Work out the finished part from the listing and answer in its coordinate system (mm). A direction names the side the tool comes from. Round coordinates to 2 decimals unless told otherwise and drop trailing zeros. Order: outer loops, then holes, each group sorted by start corner. A loop starts at its lowest first (then second) coordinate and runs counter-clockwise, first axis right, second up. Notation, with made-up numbers: (41.5, 30) - (59.5, 30) arc R17 ccw to (59.5, 53) - close; hole circle Ø6 at (-23, 82.25). An arc over 180 degrees is marked (long way). Use one line per item in the form item = value. Start each with the question number.
Q1. The part is cut by section B-B on x = 3.5. Determine the outline of the cut face in (y, z), plus the area to 3 significant figures.
Q2. The part is cut by section D-D on y = 8. Determine the outline of the cut face in (x, z), plus the area to 3 significant figures.
Q3. Given P1, Ø1.3, axis at y = -6.5, z = -16, coming from the -X side; P2, Ø2, axis at x = 13, z = -14.5, coming from the -Y side; P3, Ø2.5, axis at x = 5, y = 6.5, coming from the -Z side, each flat-ended and moving along its own axis, determine where each tip first touches the part or whether it passes through.
Q4. For a pull along X with two mould halves and no side action, classify faces 1 (the flat face through (-1, 1, 18)), 2 (the flat face through (37.42, 3.47, 8.53)), 3 (the cylindrical face through (36.579, 0.76, 14.655)) as +X half, -X half, draft (parallel to the pull), parting line (faces both ways), or undercut.
Q5. The part is cut by section A-A on x = 37.5. Determine the outline of the cut face in (y, z).
Q6. Find the intervals of material crossed by line 1 (X direction, y = 0.85, z = 15.5); line 2 (Z direction, x = -37.5, y = 0.55); line 3 (X direction, y = 4.25, z = 6), in increasing order. Write a range as [from, to].
Q7. Which of the six approach directions +Z, -Z, +X, -X, +Y, -Y give full straight-line access (tool end or side, diameter ignored) to faces 4 (the flat face through (1, 6, -12.3)), 5 (the flat face through (-13, -9, -17.5)), 6 (the flat face through (-35.05, 6, 0)), 7 (the flat face through (0, 6, 12.9))?
Q8. The part is cut by section C-C on z = 2.5. Determine the outline of the cut face in (x, y), plus the area to 3 significant figures.
from build123d import *

# Parameters (mm, degrees)
SCHIZZO1_W                   = 80
SCHIZZO1_H                   = 36
ESTRUSIONE_ESTRUSIONE1_DEPTH = 1.5
SCHIZZO2_R                   = 1.25
TAGLIO_ESTRUSIONE1_DEPTH     = 1.5
ESTRUSIONE_ESTRUSIONE2_DEPTH = 8.6
SCHIZZO3_3_W                 = 71.2
SCHIZZO3_3_H                 = 25.2
ESTRUSIONE_ESTRUSIONE3_DEPTH = 4
SCHIZZO4_W                   = 41
SCHIZZO4_H                   = 2.54
ESTRUSIONE_ESTRUSIONE4_DEPTH = 18


with BuildPart() as part:
    # Schizzo1 → Estrusione-Estrusione1 (new body)
    with BuildSketch(Plane(origin=(0, 0, 0), x_dir=(1, 0, 0), z_dir=(0, 1, 0))):
        Rectangle(SCHIZZO1_W, SCHIZZO1_H)
    extrude(amount=ESTRUSIONE_ESTRUSIONE1_DEPTH)

    # Schizzo2 → Taglio-Estrusione1 (cut)
    with BuildSketch(Plane(origin=(0, 1.5, 0), x_dir=(1, 0, 0), z_dir=(0, 1, 0))):
        with Locations((-37.5, 15.5)):
            Circle(SCHIZZO2_R)
        with Locations((37.5, 15.5)):
            Circle(SCHIZZO2_R)
        with Locations((-37.5, -15.5)):
            Circle(SCHIZZO2_R)
        with Locations((37.5, -15.5)):
            Circle(SCHIZZO2_R)
    extrude(amount=-TAGLIO_ESTRUSIONE1_DEPTH, mode=Mode.SUBTRACT)

    # Schizzo3 → Estrusione-Estrusione2 (add)
    with BuildSketch(Plane(origin=(0, 1.5, 0), x_dir=(1, 0, 0), z_dir=(0, 1, 0))):
        Polygon((36.15, 12.3), (-35.05, 12.3), (-35.05, -12.9), (36.15, -12.9), (36.15, -9.8), (36.15, -0.3), (36.15, 9.2), align=None)
    extrude(amount=ESTRUSIONE_ESTRUSIONE2_DEPTH)

    # Schizzo3_3 → Estrusione-Estrusione3 (add)
    with BuildSketch(Plane(origin=(0, 1.5, 0), x_dir=(1, 0, 0), z_dir=(0, 1, 0))):
        with Locations((0.55, -0.3)):
            Rectangle(SCHIZZO3_3_W, SCHIZZO3_3_H)
        Polygon((38.65, 6.7), (38.65, -7.3), (36.15, -9.8), (36.15, -0.3), (36.15, 9.2), align=None)
    extrude(amount=ESTRUSIONE_ESTRUSIONE3_DEPTH)

    # Schizzo4 → Estrusione-Estrusione4 (add)
    with BuildSketch(Plane.XZ):
        with Locations((-12.5, -16.23)):
            Rectangle(SCHIZZO4_W, SCHIZZO4_H)
    extrude(amount=ESTRUSIONE_ESTRUSIONE4_DEPTH)


solid = part.part
Found:
q1.outline = (-18, -17.5) - (0, -17.5) - (0, -18) - (1.5, -18) - (1.5, -12.3) - (10.1, -12.3) - (10.1, 12.9) - (1.5, 12.9) - (1.5, 18) - (0, 18) - (0, -14.96) - (-18, -14.96) - close
q1.area = 316 mm²
q2.outline = (-35.05, -12.3) - (36.15, -12.3) - (36.15, 12.9) - (-35.05, 12.9) - close
q2.area = 1,790 mm²
q3.P1 = -33
q3.P2 = 0
q3.P3 = -12.3
q4.face_1 = draft
q4.face_2 = +X half
q4.face_3 = undercut
q5.outline = (0, -18) - (1.5, -18) - (1.5, -16.75) - (0, -16.75) - close; (0, -14.25) - (1.5, -14.25) - (1.5, -7.85) - (5.5, -7.85) - (5.5, 8.45) - (1.5, 8.45) - (1.5, 14.25) - (0, 14.25) - close; (0, 16.75) - (1.5, 16.75) - (1.5, 18) - (0, 18) - close
q6.line_1 = [-40, -38.75], [-36.25, 36.25], [38.75, 40]
q6.line_2 = [-18, -16.75], [-14.25, 14.25], [16.75, 18]
q6.line_3 = [-35.05, 38.65]
q7.face_4 = -Z, +X, -X, +Y
q7.face_5 = -Z, +X, -X, -Y
q7.face_6 = +Z, -Z, -X, +Y
q7.face_7 = +Z, +X, -X, +Y
q8.outline = (-40, 0) - (40, 0) - (40, 1.5) - (38.65, 1.5) - (38.65, 5.5) - (36.15, 5.5) - (36.15, 10.1) - (-35.05, 10.1) - (-35.05, 1.5) - (-40, 1.5) - close
q8.area = 742 mm²
